The model under review builds one solid part; all positions refer to its coordinate system, in mm. A direction names the side the tool comes from. Round coordinates to 2 decimals unless told otherwise and drop trailing zeros. Write each loop counter-clockwise with the first axis right and the second up, starting at its lowest first coordinate (ties: lowest second). Pieces come first, ordered by that corner, then holes. Notation, with made-up numbers: (69.5, -29.75) - (104.5, -29.75) arc R36 ccw to (104.5, 7.25) - close; hole circle Ø8 at (75, -7). An arc over 180 degrees is marked (long way). Use one line per item in the form item = value.
from build123d import *

# Parameters (mm, degrees)
SKETCH_1_W          = 50
SKETCH_1_H          = 100
EXTRUDE_1_DEPTH     = 5
SKETCH_2_W          = 29.5
SKETCH_2_H          = 2.4
EXTRUDE_2_DEPTH     = 7
SKETCH_3_W          = 29.5
SKETCH_3_H          = 2.4
EXTRUDE_3_DEPTH     = 7
CUT_EXTRUDE_1_DEPTH = 5
FILLET_1_R          = 3
SKETCH_5_R          = 1.5
CUT_EXTRUDE_2_DEPTH = 5.9
SKETCH_6_R          = 1.5
CUT_EXTRUDE_3_DEPTH = 5.9


with BuildPart() as part:
    # 草图1 → 凸台-拉伸1 (new body)
    with BuildSketch(Plane.XY):
        Rectangle(SKETCH_1_W, SKETCH_1_H)
    extrude(amount=-EXTRUDE_1_DEPTH)

    # 草图2 → 凸台-拉伸2 (add)
    with BuildSketch(Plane(origin=(0, 50, 0), x_dir=(1, 0, 0), z_dir=(0, 1, 0))):
        with Locations((0, 3.7)):
            Rectangle(SKETCH_2_W, SKETCH_2_H)
        with Locations((0, 1.3)):
            Rectangle(SKETCH_2_W, SKETCH_2_H)
    extrude(amount=EXTRUDE_2_DEPTH)

    # 草图3 → 凸台-拉伸3 (add)
    with BuildSketch(Plane.XZ.offset(50)):
        with Locations((0, -1.3)):
            Rectangle(SKETCH_3_W, SKETCH_3_H)
        with Locations((0, -3.7)):
            Rectangle(SKETCH_3_W, SKETCH_3_H)
    extrude(amount=EXTRUDE_3_DEPTH)

    # 草图4 → 切除-拉伸1 (cut)
    with BuildSketch(Plane.XY):
        with BuildLine():
            Line((0, 20), (0, 24))
            Line((0, 24), (-15, 24))
            ThreePointArc((-15, 24), (-17.828427125, 22.828427125), (-19, 20))
            Line((-19, 20), (0, 20))
        make_face()
        with BuildLine():
            Line((15, 24), (0, 24))
            Line((0, 24), (0, 20))
            Line((0, 20), (19, 20))
            ThreePointArc((19, 20), (17.828427125, 22.828427125), (15, 24))
        make_face()
        with BuildLine():
            Line((0, 16), (0, 20))
            Line((0, 20), (-19, 20))
            ThreePointArc((-19, 20), (-17.828427125, 17.171572875), (-15, 16))
            Line((-15, 16), (0, 16))
        make_face()
        with BuildLine():
            Line((19, 20), (0, 20))
            Line((0, 20), (0, 16))
            Line((0, 16), (15, 16))
            ThreePointArc((15, 16), (17.828427125, 17.171572875), (19, 20))
        make_face()
        with BuildLine():
            Line((0, 0), (0, 4))
            Line((0, 4), (-15, 4))
            ThreePointArc((-15, 4), (-17.828427125, 2.828427125), (-19, 0))
            Line((-19, 0), (0, 0))
        make_face()
        with BuildLine():
            Line((15, 4), (0, 4))
            Line((0, 4), (0, 0))
            Line((0, 0), (19, 0))
            ThreePointArc((19, 0), (17.828427125, 2.828427125), (15, 4))
        make_face()
        with BuildLine():
            Line((0, -4), (0, 0))
            Line((0, 0), (-19, 0))
            ThreePointArc((-19, 0), (-17.828427125, -2.828427125), (-15, -4))
            Line((-15, -4), (0, -4))
        make_face()
        with BuildLine():
            Line((19, 0), (0, 0))
            Line((0, 0), (0, -4))
            Line((0, -4), (15, -4))
            ThreePointArc((15, -4), (17.828427125, -2.828427125), (19, 0))
        make_face()
        with BuildLine():
            Line((0, -20), (0, -16))
            Line((0, -16), (-15, -16))
            ThreePointArc((-15, -16), (-17.828427125, -17.171572875), (-19, -20))
            Line((-19, -20), (0, -20))
        make_face()
        with BuildLine():
            Line((0, -24), (0, -20))
            Line((0, -20), (-19, -20))
            ThreePointArc((-19, -20), (-17.828427125, -22.828427125), (-15, -24))
            Line((-15, -24), (0, -24))
        make_face()
        with BuildLine():
            Line((15, -16), (0, -16))
            Line((0, -16), (0, -20))
            Line((0, -20), (19, -20))
            ThreePointArc((19, -20), (17.828427125, -17.171572875), (15, -16))
        make_face()
        with BuildLine():
            Line((19, -20), (0, -20))
            Line((0, -20), (0, -24))
            Line((0, -24), (15, -24))
            ThreePointArc((15, -24), (17.828427125, -22.828427125), (19, -20))
        make_face()
    extrude(amount=-CUT_EXTRUDE_1_DEPTH, mode=Mode.SUBTRACT)

    # 圆角1
    fillet_1_edges = [part.edges().sort_by_distance(p)[0] for p in [
        (14.75, 57, -2.5),
        (-14.75, 57, -2.5),
        (14.75, -57, -2.5),
        (-14.75, -57, -2.5),
    ]]
    fillet(fillet_1_edges, radius=FILLET_1_R)

    # 草图5 → 切除-拉伸2 (cut, through all)
    with BuildSketch(Plane.XY.offset(-0.1)):
        with Locations((0, 53.5)):
            Circle(SKETCH_5_R)
    extrude(amount=-CUT_EXTRUDE_2_DEPTH, mode=Mode.SUBTRACT)

    # 草图6 → 切除-拉伸3 (cut, through all)
    with BuildSketch(Plane.XY.offset(-0.1)):
        with Locations((0, -53.5)):
            Circle(SKETCH_6_R)
    extrude(amount=-CUT_EXTRUDE_3_DEPTH, mode=Mode.SUBTRACT)


solid = part.part
(1) Machinability: for faces 1 (the flat face through (0, 4, -2)), 2 (the flat face through (14.75, 52, -2)), 3 (the flat face through (-14.75, -52, -2)), 4 (the flat face through (0, -51, -0.1)), 5 (the flat face through (-14.75, 52, -3)), which of the approach directions +Z, -Z, +X, -X, +Y, -Y give a long, thin tool a straight path to every point of the face, cutting with its end or side? Answer none if there is none.
Geometry results:
face_1 = +Z, -Z
face_2 = +Z, -Z, +X, +Y
face_3 = +Z, -Z, -X, -Y
face_4 = +Z, +X, -X, -Y
face_5 = +Z, -Z, -X, +Y
(2) The part is to be moulded in two halves that separate along Y. For faces 6 (the flat face through (0, -4, -2)), 7 (the cylindrical face through (13.89, 56.1, -2.53)), 8 (the cylindrical face through (-13.89, -56.1, -2.53)), say which applies: +Y half, -Y half, draft (parallel to the pull), parting line (faces both ways), or undercut.
Geometry results:
face_6 = undercut
face_7 = +Y half
face_8 = -Y half
(3) Insertion check: P1, Ø2.5, axis at x = 0, y = 53.5, coming from the -Z side; P2, Ø10, axis at x = -6.5, y = -5.5, coming from the +Z side; P3, Ø1.2, axis at y = 52, z = -2.5, coming from the +X side; P4, Ø3.5, axis at x = -1, y = -53, coming from the -Z side. Each pin has a flat end and moves straight along its axis. Give the tip position at first contact, or say it passes through.
Geometry results:
P1 = through
P2 = 0
P3 = 14.75
P4 = -4.9
(4) Add section B-B on x = 0. Count the separate pieces of the cut face and the enclosed holes in it, then the cut area to 3 significant figures.
Geometry results:
separate_pieces = 6
enclosed_holes = 0
area = 418 mm2
(5) To check wall thickness, follow L1, parallel to Y at x = 4, z = -3.4; L2, parallel to Y at x = 0, z = -3.5; L3, parallel to Y at x = -15, z = -4.55. State the ranges of each line that lie inside material, in increasing order.
Geometry results:
L1 = -57 to -24, -16 to -4, 4 to 16, 24 to 57
L2 = -57 to -55, -52 to -24, -16 to -4, 4 to 16, 24 to 52, 55 to 57
L3 = -50 to -24, -16 to -4, 4 to 16, 24 to 50
(6) Add section A-A on x = 6.5. Write out the cut boundary in (y, z), then the cut area to 3 significant figures.
Geometry results:
outline = (-57, -4.9) - (-50, -4.9) - (-50, -5) - (-24, -5) - (-24, 0) - (-50, 0) - (-50, -0.1) - (-57, -0.1) - close; (-16, -5) - (-4, -5) - (-4, 0) - (-16, 0) - close; (4, -5) - (16, -5) - (16, 0) - (4, 0) - close; (24, -5) - (50, -5) - (50, -4.9) - (57, -4.9) - (57, -0.1) - (50, -0.1) - (50, 0) - (24, 0) - close
area = 447 mm2
(7) Add section C-C on y = -22.5. Write out the cut boundary in (x, z), then the cut area to 3 significant figures.
Geometry results:
outline = (-25, -5) - (-18.12, -5) - (-18.12, 0) - (-25, 0) - close; (18.12, -5) - (25, -5) - (25, 0) - (18.12, 0) - close
area = 68.8 mm2
